For this review, take the finished solid that the model builds, in its own axes (mm). A direction names the side the tool comes from. Coordinates: 2 decimals unless noted, no trailing zeros. Loops run counter-clockwise (first coordinate to the right, second up) from the corner with the lowest first, then second, coordinate; pieces in that order, holes last.
```python
from build123d import *

# Parameters (mm, degrees)
F0_W     = 30
F0_H     = 44
F0_R     = 1.562
F1_DEPTH = 1.5
F2_W     = 30
F2_H     = 2
F3_DEPTH = 7
F4_W     = 30
F4_H     = 2
F5_DEPTH = 2
F6_W     = 30
F6_H     = 2
F7_DEPTH = 2


with BuildPart() as f1:
    # F0 (on Front) → F1 (new body, symmetric)
    with BuildSketch(Plane.XZ):
        Rectangle(F0_W, F0_H)
        Circle(F0_R, mode=Mode.SUBTRACT)
    extrude(amount=F1_DEPTH, both=True)

    # F2 (on face) → F3 (join)
    with BuildSketch(Plane.XZ.offset(1.5)):
        with Locations((0, 21)):
            Rectangle(F2_W, F2_H)
        with Locations((0, -21)):
            Rectangle(F2_W, F2_H)
    extrude(amount=F3_DEPTH)

    # F4 (on face) → F5 (join)
    with BuildSketch(Plane(origin=(0, 0, 20), x_dir=(1, 0, 0), z_dir=(0, 0, -1))):
        with Locations((0, 7.5)):
            Rectangle(F4_W, F4_H)
    extrude(amount=F5_DEPTH)

    # F6 (on face) → F7 (join)
    with BuildSketch(Plane.XY.offset(-20)):
        with Locations((0, -7.5)):
            Rectangle(F6_W, F6_H)
    extrude(amount=F7_DEPTH)


solid = f1.part
```
Q1. Consider section A-A (z = 0). State the section outline as (x, y) points, then the cut area to 3 significant figures.
Q2. The part is to be moulded in two halves that separate along X. For faces 1 (the face through (15, -1, 0)), 2 (the face through (-15, -1, 0)), 3 (the face through (0, -4, 20)), 4 (the face through (-0.2, 0.02, 1.55)), say which applies: +X half, -X half, draft (parallel to the pull), parting line (faces both ways), or undercut.
Q3. Wall thickness on probe 1 along Z at (x, y) = (-0.25, -2.25); probe 2 along Z at (x, y) = (0, -0.7); probe 3 along Y at (x, z) = (-1.5, 2.5): over which ranges is each line inside the solid? List them lowest first.
Q4. Consider section B-B (y = -4). State the section outline as (x, z) points, then the cut area to 3 significant figures.
Q5. Machinability: for faces 5 (the face through (0, -8.5, 20)), 6 (the face through (0, -4, -20)), 7 (the face through (0, -8, 18)), which of the approach directions +Z, -Z, +X, -X, +Y, -Y give a long, thin tool a straight path to every point of the face, cutting with its end or side? Answer none if there is none.
Q6. Consider section C-C (x = 0). State the section outline as (y, z) points.
Q7. Consider section D-D (x = 4.5). State the section outline as (y, z) points.
Model answer:
1. outline: (-15, -1.5) - (-1.56, -1.5) - (-1.56, 1.5) - (-15, 1.5) - close; (1.56, -1.5) - (15, -1.5) - (15, 1.5) - (1.56, 1.5) - close
1. area: 80.6 mm2
2. face 1: +X half
2. face 2: -X half
2. face 3: draft
2. face 4: undercut
3. probe 1: z = -22 to -20, 20 to 22
3. probe 2: z = -22 to -1.56, 1.56 to 22
3. probe 3: y = -1.5 to 1.5
4. outline: (-15, -22) - (15, -22) - (15, -20) - (-15, -20) - close; (-15, 20) - (15, 20) - (15, 22) - (-15, 22) - close
4. area: 120 mm2
5. face 5: +Z, -Z, +X, -X, -Y
5. face 6: +X, -X
5. face 7: +X, -X, -Y
6. outline: (-8.5, -22) - (1.5, -22) - (1.5, -1.56) - (-1.5, -1.56) - (-1.5, -20) - (-6.5, -20) - (-6.5, -18) - (-8.5, -18) - close; (-8.5, 18) - (-6.5, 18) - (-6.5, 20) - (-1.5, 20) - (-1.5, 1.56) - (1.5, 1.56) - (1.5, 22) - (-8.5, 22) - close
7. outline: (-8.5, -22) - (1.5, -22) - (1.5, 22) - (-8.5, 22) - (-8.5, 18) - (-6.5, 18) - (-6.5, 20) - (-1.5, 20) - (-1.5, -20) - (-6.5, -20) - (-6.5, -18) - (-8.5, -18) - close
